```python
from build123d import *

# Parameters (mm, degrees)
MAIN_DEPTH                 = 20
ESQUISSE2_R                = 1.6
TOPHOLE_DEPTH              = 5
R_P_TITION_LIN_AIRE1_COUNT = 2
R_P_TITION_LIN_AIRE1_PITCH = 10


with BuildPart() as part:
    # Esquisse1 → Main (new body)
    with BuildSketch(Plane.XY):
        Polygon((-5, 0), (-5, 3), (-1.45, 3), (-1.45, 4), (1.45, 4), (1.45, 3), (5, 3), (5, 0), align=None)
    main = extrude(amount=MAIN_DEPTH)

    # Esquisse2 → TopHole (cut, through all)
    with BuildSketch(Plane(origin=(0, 4, 0), x_dir=(1, 0, 0), z_dir=(0, 1, 0))):
        with Locations((0, -5)):
            Circle(ESQUISSE2_R)
        with Locations((0, -15)):
            Circle(ESQUISSE2_R)
    tophole = extrude(amount=-TOPHOLE_DEPTH, mode=Mode.SUBTRACT)

    # Répétition linéaire1: Main, TopHole ×2
    with Locations(*[(-i * R_P_TITION_LIN_AIRE1_PITCH, 0, 0) for i in range(1, R_P_TITION_LIN_AIRE1_COUNT)]):
        add(main)
        add(tophole, mode=Mode.SUBTRACT)


solid = part.part
```
Geometry: final body of the model. Coordinates: model frame, mm. A direction names the side the tool comes from. Give positions to 0.01 mm unless a question says otherwise; leave off trailing zeros. Order: outer loops, then holes, each group sorted by start corner. A loop starts at its lowest first (then second) coordinate and runs counter-clockwise, first axis right, second up. Notation, with made-up numbers: (3.25, -33) -> (23.25, -33) arc R21 ccw to (23.25, 4) -> close; hole circle Ø7 at (25, 34.25). An arc over 180 degrees is marked (long way). Write each question's results on one line, items separated by ' | '. Start each with the question number.
1) Line query: line 1 (Z direction, x = 0, y = 1.45); line 2 (X direction, y = 1.25, z = 15); line 3 (Z direction, x = -8.75, y = 1.25). Output: solid intervals per line, ascending. Write a range as from..to.
2) Section C-C (x = 0). Return loops of the section in (y, z).
3) Draft query along Z for faces 5 (the cylindrical face through (-1.6, 2.03, 14.93)), 6 (the flat face through (0, 4, 10)), 7 (the flat face through (-5, 2, 0)). Return one class per face: pulls with the +Z half, pulls with the -Z half, needs draft (parallel to the pull), parting line crosses it, or undercut.
4) Set-up query: faces 1 (the flat face through (1.45, 3.5, 17.8)), 2 (the flat face through (-11.45, 3.5, 2.1)), 3 (the flat face through (-15, 1, 10)), 4 (the flat face through (-5, 3, 10)). Return all of +Z, -Z, +X, -X, +Y, -Y with unobstructed straight access to the full face (end or side cutting, diameter ignored); none if empty.
5) Section A-A (z = 5). Return loops of the section in (x, y), then the cut area to 3 significant figures.
6) Section D-D (y = 1.55). Return loops of the section in (x, z), then the cut area to 3 significant figures.
7) First-contact query: pin 1 (0.8 mm diameter, centred on y = 3.5, z = 17.5, fed in from -X); pin 2 (1.8 mm diameter, centred on x = 4, z = 9.5, fed in from +Y); pin 3 (0.8 mm diameter, centred on y = 3.5, z = 9.5, fed in from +X). Flat tips, straight axial feed; report the tip coordinate or a pass-through.
8) Section B-B (y = 3.45). Return loops of the section in (x, z).
Calculated:
1) line 1: 0..3.4, 6.6..13.4, 16.6..20 | line 2: -15..-11.6, -8.4..-1.6, 1.6..5 | line 3: 0..4, 6..14, 16..20
2) outline: (0, 0) -> (4, 0) -> (4, 3.4) -> (0, 3.4) -> close; (0, 6.6) -> (4, 6.6) -> (4, 13.4) -> (0, 13.4) -> close; (0, 16.6) -> (4, 16.6) -> (4, 20) -> (0, 20) -> close
3) face 5: undercut | face 6: needs draft | face 7: pulls with the -Z half
4) face 1: +Z, -Z, +X, +Y | face 2: +Z, -Z, -X, +Y | face 3: +Z, -Z, -X, +Y, -Y | face 4: +Z, -Z, +Y
5) outline: (-15, 0) -> (-11.6, 0) -> (-11.6, 3) -> (-15, 3) -> close; (-8.4, 0) -> (-1.6, 0) -> (-1.6, 3) -> (-8.4, 3) -> close; (1.6, 0) -> (5, 0) -> (5, 3) -> (1.6, 3) -> close | area: 40.8 mm2
6) outline: (-15, 0) -> (5, 0) -> (5, 20) -> (-15, 20) -> close; hole circle Ø3.2 at (-10, 5); hole circle Ø3.2 at (-10, 15); hole circle Ø3.2 at (0, 5); hole circle Ø3.2 at (0, 15) | area: 368 mm2
7) pin 1: x = -11.45 | pin 2: y = 3 | pin 3: x = 1.45
8) outline: (-11.45, 0) -> (-8.55, 0) -> (-8.55, 4.32) arc R1.6 cw to (-11.45, 4.32) -> close; (-11.45, 5.68) arc R1.6 cw to (-8.55, 5.68) -> (-8.55, 14.32) arc R1.6 cw to (-11.45, 14.32) -> close; (-11.45, 15.68) arc R1.6 cw to (-8.55, 15.68) -> (-8.55, 20) -> (-11.45, 20) -> close; (-1.45, 0) -> (1.45, 0) -> (1.45, 4.32) arc R1.6 cw to (-1.45, 4.32) -> close; (-1.45, 5.68) arc R1.6 cw to (1.45, 5.68) -> (1.45, 14.32) arc R1.6 cw to (-1.45, 14.32) -> close; (-1.45, 15.68) arc R1.6 cw to (1.45, 15.68) -> (1.45, 20) -> (-1.45, 20) -> close
